Source: CAD feature listing. Evaluate the final solid. Frame: model axes, mm. A direction names the side the tool comes from. Coordinates: 2 decimals unless noted, no trailing zeros. Write each loop counter-clockwise with the first axis right and the second up, starting at its lowest first coordinate (ties: lowest second). Pieces come first, ordered by that corner, then holes. Notation, with made-up numbers: (-10, 89) -> (34, 89) arc R10 cw to (34, 93) -> close; hole circle Ø6 at (79, 82.25). An arc over 180 degrees is marked (long way). Write item = value, one per line.
from build123d import *

# Parameters (mm, degrees)
SKETCH1_W           = 26.9875
SKETCH1_H           = 26.9875
BOSS_EXTRUDE1_DEPTH = 2.38125
SKETCH2_W           = 6.35
SKETCH2_H           = 6.35
CUT_EXTRUDE1_DEPTH  = 20.231040785
SKETCH3_R           = 1.27
CUT_EXTRUDE2_DEPTH  = 20.231040785
CUT_EXTRUDE3_DEPTH  = 1.5875
FILLET1_R           = 1.5875
FILLET2_R           = 1.5875


with BuildPart() as part:
    # Sketch1 → Boss-Extrude1 (new body)
    with BuildSketch(Plane(origin=(0, 0, 0), x_dir=(1, 0, 0), z_dir=(0, 1, 0))):
        Rectangle(SKETCH1_W, SKETCH1_H)
    extrude(amount=BOSS_EXTRUDE1_DEPTH)

    # Sketch2 → Cut-Extrude1 (cut, through all)
    with BuildSketch(Plane(origin=(0, 2.38125, 0), x_dir=(1, 0, 0), z_dir=(0, 1, 0))):
        Rectangle(SKETCH2_W, SKETCH2_H)
    extrude(amount=-CUT_EXTRUDE1_DEPTH, mode=Mode.SUBTRACT)

    # Sketch3 → Cut-Extrude2 (cut, through all)
    with BuildSketch(Plane(origin=(0, 2.38125, 0), x_dir=(1, 0, 0), z_dir=(0, 1, 0))):
        with Locations(Location((-10.16, 10.16, 0), (0, 0, 270))):
            Circle(SKETCH3_R)
        with Locations(Location((10.16, 10.16, 0), (0, 0, 270))):
            Circle(SKETCH3_R)
        with Locations(Location((10.16, -10.16, 0), (0, 0, 270))):
            Circle(SKETCH3_R)
        with Locations(Location((-10.16, -10.16, 0), (0, 0, 270))):
            Circle(SKETCH3_R)
    extrude(amount=-CUT_EXTRUDE2_DEPTH, mode=Mode.SUBTRACT)

    # Sketch4 → Cut-Extrude3 (cut)
    with BuildSketch(Plane(origin=(0, 2.38125, 0), x_dir=(1, 0, 0), z_dir=(0, 1, 0))):
        with BuildLine():
            Line((-11.90625, -7.131243036), (-11.90625, 7.131243036))
            ThreePointArc((-11.90625, 7.131243036), (-11.582088833, 7.771184744), (-10.874375, 7.888432277))
            ThreePointArc((-10.874375, 7.888432277), (-8.259382698, 8.725424998), (-8.171264167, 11.4696875))
            ThreePointArc((-8.171264167, 11.4696875), (-8.207122766, 12.282758684), (-7.508352222, 12.7))
            Line((-7.508352222, 12.7), (7.508352222, 12.7))
            ThreePointArc((7.508352222, 12.7), (8.207122766, 12.282758684), (8.171264167, 11.4696875))
            ThreePointArc((8.171264167, 11.4696875), (8.259382698, 8.725424998), (10.874375, 7.888432277))
            ThreePointArc((10.874375, 7.888432277), (11.582088833, 7.771184744), (11.90625, 7.131243036))
            Line((11.90625, 7.131243036), (11.90625, -7.131243036))
            ThreePointArc((11.90625, -7.131243036), (11.582088833, -7.771184744), (10.874375, -7.888432277))
            ThreePointArc((10.874375, -7.888432277), (8.259382698, -8.725424998), (8.171264167, -11.4696875))
            ThreePointArc((8.171264167, -11.4696875), (8.207122766, -12.282758684), (7.508352222, -12.7))
            Line((7.508352222, -12.7), (-7.508352222, -12.7))
            ThreePointArc((-7.508352222, -12.7), (-8.207122766, -12.282758684), (-8.171264167, -11.4696875))
            ThreePointArc((-8.171264167, -11.4696875), (-8.259382698, -8.725424998), (-10.874375, -7.888432277))
            ThreePointArc((-10.874375, -7.888432277), (-11.582088833, -7.771184744), (-11.90625, -7.131243036))
        make_face()
    extrude(amount=-CUT_EXTRUDE3_DEPTH, mode=Mode.SUBTRACT)

    # Fillet1
    fillet1_edges = [part.edges().sort_by_distance(p)[0] for p in [
        (13.49375, 1.190625, 13.49375),
        (-13.49375, 1.190625, 13.49375),
        (-13.49375, 1.190625, -13.49375),
        (13.49375, 1.190625, -13.49375),
    ]]
    fillet(fillet1_edges, radius=FILLET1_R)

    # Fillet2
    fillet2_edges = [part.edges().sort_by_distance(p)[0] for p in [
        (13.49375, 0, 0),
        (0, 0, 13.49375),
        (-13.49375, 0, 0),
        (0, 0, -13.49375),
        (-13.028782015, 0, 13.028782015),
        (-13.028782015, 0, -13.028782015),
        (13.028782015, 0, -13.028782015),
        (13.028782015, 0, 13.028782015),
    ]]
    fillet(fillet2_edges, radius=FILLET2_R)


solid = part.part
1) Pull-direction query (X, two-part tool) for faces 1 (the cylindrical face through (8.201, 1.599, -12.293)), 2 (the cylindrical face through (13.02, 1.99, 13.04)), 3 (the flat face through (-12.1, 2.381, -0.1)); classes: +X half, -X half, draft (parallel to the pull), parting line (faces both ways), or undercut.
Answer block:
face_1 = undercut
face_2 = +X half
face_3 = draft
2) Cut plane B-B, the plane x = -0.75. Output: boundary loops of the cut face in (y, z) (1 decimal).
Answer block:
outline = (0, -11.9) arc R1.6 ccw to (1.6, -13.5) -> (2.4, -13.5) -> (2.4, -12.7) -> (0.8, -12.7) -> (0.8, -3.2) -> (0, -3.2) -> close; (0, 3.2) -> (0.8, 3.2) -> (0.8, 12.7) -> (2.4, 12.7) -> (2.4, 13.5) -> (1.6, 13.5) arc R1.6 ccw to (0, 11.9) -> close
3) First-contact query: pin 1 Ø0.6 at (x, y) = (-1, 0.5) entering from +Z; pin 2 Ø7 at (x, z) = (4, -0.5) entering from +Y; pin 3 Ø1.5 at (x, z) = (10.16, -10.16) entering from -Y; pin 4 Ø0.9 at (x, y) = (0, 0.5) entering from -Z. Flat tips, straight axial feed; report the tip coordinate or a pass-through.
Answer block:
pin_1 = 13.28
pin_2 = 0.79
pin_3 = through
pin_4 = -13.36
4) Cut plane A-A, the plane z = -10.16. Output: boundary loops of the cut face in (x, y) (1 decimal).
Answer block:
outline = (-13.5, 1.6) arc R1.6 ccw to (-11.9, 0) -> (-11.4, 0) -> (-11.4, 2.4) -> (-13.5, 2.4) -> close; (-8.9, 0) -> (8.9, 0) -> (8.9, 2.4) -> (7.8, 2.4) -> (7.8, 0.8) -> (-7.8, 0.8) -> (-7.8, 2.4) -> (-8.9, 2.4) -> close; (11.4, 0) -> (11.9, 0) arc R1.6 ccw to (13.5, 1.6) -> (13.5, 2.4) -> (11.4, 2.4) -> close
5) Cut plane C-C, the plane x = -10.16. Output: boundary loops of the cut face in (y, z) (1 decimal).
Answer block:
outline = (0, -11.9) arc R1.6 ccw to (1.6, -13.5) -> (2.4, -13.5) -> (2.4, -11.4) -> (0, -11.4) -> close; (0, -8.9) -> (2.4, -8.9) -> (2.4, -7.8) -> (0.8, -7.8) -> (0.8, 7.8) -> (2.4, 7.8) -> (2.4, 8.9) -> (0, 8.9) -> close; (0, 11.4) -> (2.4, 11.4) -> (2.4, 13.5) -> (1.6, 13.5) arc R1.6 ccw to (0, 11.9) -> close
6) Reachability of faces 4 (the cylindrical face through (9.67, 1.21, -8.99)), 5 (the cylindrical face through (11.57, 1.6, -7.78)) from +Z, -Z, +X, -X, +Y, -Y: full face, straight path, thin tool, end or side. Return the list, or none.
Answer block:
face_4 = +Y, -Y
face_5 = +Y
7) Cut plane D-D, the plane z = -0.75. Output: boundary loops of the cut face in (x, y) (1 decimal).
Answer block:
outline = (-13.5, 1.6) arc R1.6 ccw to (-11.9, 0) -> (-3.2, 0) -> (-3.2, 0.8) -> (-11.9, 0.8) -> (-11.9, 2.4) -> (-13.5, 2.4) -> close; (3.2, 0) -> (11.9, 0) arc R1.6 ccw to (13.5, 1.6) -> (13.5, 2.4) -> (11.9, 2.4) -> (11.9, 0.8) -> (3.2, 0.8) -> close
8) Material intervals for probe 1 along X at (y, z) = (1.7, 10.16); probe 2 along Z at (x, y) = (1.75, 2.15); probe 3 along X at (y, z) = (0.9, -10.16), sorted ascending. Write a range as [from, to].
Answer block:
probe_1 = [-13.49, -11.43], [-8.89, -7.78], [7.78, 8.89], [11.43, 13.49]
probe_2 = [-13.49, -12.7], [12.7, 13.49]
probe_3 = [-13.34, -11.43], [-8.89, -7.78], [7.78, 8.89], [11.43, 13.34]
